Verification items for the finished model (mm, model axes). Round coordinates to 2 decimals unless told otherwise and drop trailing zeros. Loops run counter-clockwise (first coordinate to the right, second up) from the corner with the lowest first, then second, coordinate; pieces in that order, holes last.
from build123d import *

# Parameters (mm, degrees)
SKETCH1_R           = 9.625
BOSS_EXTRUDE1_DEPTH = 0.6


with BuildPart() as part:
    # Sketch1 → Boss-Extrude1 (new body)
    with BuildSketch(Plane(origin=(0, 0, 0), x_dir=(1, 0, 0), z_dir=(0, 1, 0))):
        with BuildLine():
            ThreePointArc((13.474991136, 1.1), (13.700677051, 0.553298036), (14.246293378, 0.325))
            ThreePointArc((14.246293378, 0.325), (13.165283338, 5.453238911), (10.303460358, 9.84384095))
            ThreePointArc((10.303460358, 9.84384095), (9.29660086, 9.429085476), (8.290823601, 9.846458519))
            ThreePointArc((8.290823601, 9.846458519), (8.290823601, 10.306075068), (8.750440149, 10.306075068))
            ThreePointArc((8.750440149, 10.306075068), (9.296600856, 10.079082443), (9.84384095, 10.303460358))
            ThreePointArc((9.84384095, 10.303460358), (5.453238911, 13.165283338), (0.325, 14.246293378))
            ThreePointArc((0.325, 14.246293378), (-0.09368077, 13.24105979), (-1.1, 12.824995179))
            ThreePointArc((-1.1, 12.824995179), (-1.424997978, 13.149993158), (-1.1, 13.474991136))
            ThreePointArc((-1.1, 13.474991136), (-0.553298036, 13.700677051), (-0.325, 14.246293378))
            ThreePointArc((-0.325, 14.246293378), (-5.453238911, 13.165283338), (-9.84384095, 10.303460358))
            ThreePointArc((-9.84384095, 10.303460358), (-9.429085476, 9.29660086), (-9.846458519, 8.290823601))
            ThreePointArc((-9.846458519, 8.290823601), (-10.306075068, 8.290823601), (-10.306075068, 8.750440149))
            ThreePointArc((-10.306075068, 8.750440149), (-10.079082443, 9.296600856), (-10.303460358, 9.84384095))
            ThreePointArc((-10.303460358, 9.84384095), (-13.165283338, 5.453238911), (-14.246293378, 0.325))
            ThreePointArc((-14.246293378, 0.325), (-13.24105979, -0.09368077), (-12.824995179, -1.1))
            ThreePointArc((-12.824995179, -1.1), (-13.149993158, -1.424997978), (-13.474991136, -1.1))
            ThreePointArc((-13.474991136, -1.1), (-13.700677051, -0.553298036), (-14.246293378, -0.325))
            ThreePointArc((-14.246293378, -0.325), (-13.165283338, -5.453238911), (-10.303460358, -9.84384095))
            ThreePointArc((-10.303460358, -9.84384095), (-9.29660086, -9.429085476), (-8.290823601, -9.846458519))
            ThreePointArc((-8.290823601, -9.846458519), (-8.290823601, -10.306075068), (-8.750440149, -10.306075068))
            ThreePointArc((-8.750440149, -10.306075068), (-9.296600856, -10.079082443), (-9.84384095, -10.303460358))
            ThreePointArc((-9.84384095, -10.303460358), (-5.453238911, -13.165283338), (-0.325, -14.246293378))
            ThreePointArc((-0.325, -14.246293378), (0.09368077, -13.24105979), (1.1, -12.824995179))
            ThreePointArc((1.1, -12.824995179), (1.424997978, -13.149993158), (1.1, -13.474991136))
            ThreePointArc((1.1, -13.474991136), (0.553298036, -13.700677051), (0.325, -14.246293378))
            ThreePointArc((0.325, -14.246293378), (5.453238911, -13.165283338), (9.84384095, -10.303460358))
            ThreePointArc((9.84384095, -10.303460358), (9.429085476, -9.29660086), (9.846458519, -8.290823601))
            ThreePointArc((9.846458519, -8.290823601), (10.306075068, -8.290823601), (10.306075068, -8.750440149))
            ThreePointArc((10.306075068, -8.750440149), (10.079082443, -9.296600856), (10.303460358, -9.84384095))
            ThreePointArc((10.303460358, -9.84384095), (13.165283338, -5.453238911), (14.246293378, -0.325))
            ThreePointArc((14.246293378, -0.325), (13.24105979, 0.09368077), (12.824995179, 1.1))
            ThreePointArc((12.824995179, 1.1), (13.149993158, 1.424997978), (13.474991136, 1.1))
        make_face()
        with BuildLine():
            ThreePointArc((-4.5, -11.6), (-5.1, -11), (-4.5, -10.4))
            Line((-4.5, -10.4), (4.5, -10.4))
            ThreePointArc((4.5, -10.4), (5.1, -11), (4.5, -11.6))
            Line((4.5, -11.6), (-4.5, -11.6))
        make_face(mode=Mode.SUBTRACT)
        with BuildLine():
            ThreePointArc((-11.6, 4.5), (-11, 5.1), (-10.4, 4.5))
            Line((-10.4, 4.5), (-10.4, -4.5))
            ThreePointArc((-10.4, -4.5), (-11, -5.1), (-11.6, -4.5))
            Line((-11.6, -4.5), (-11.6, 4.5))
        make_face(mode=Mode.SUBTRACT)
        with Locations(Location((0, 0, 0), (0, 0, 270))):
            Circle(SKETCH1_R, mode=Mode.SUBTRACT)
        with BuildLine():
            ThreePointArc((11.6, -4.5), (11, -5.1), (10.4, -4.5))
            Line((10.4, -4.5), (10.4, 4.5))
            ThreePointArc((10.4, 4.5), (11, 5.1), (11.6, 4.5))
            Line((11.6, 4.5), (11.6, -4.5))
        make_face(mode=Mode.SUBTRACT)
        with BuildLine():
            ThreePointArc((4.5, 11.6), (5.1, 11), (4.5, 10.4))
            Line((4.5, 10.4), (-4.5, 10.4))
            ThreePointArc((-4.5, 10.4), (-5.1, 11), (-4.5, 11.6))
            Line((-4.5, 11.6), (4.5, 11.6))
        make_face(mode=Mode.SUBTRACT)
    extrude(amount=BOSS_EXTRUDE1_DEPTH)


solid = part.part
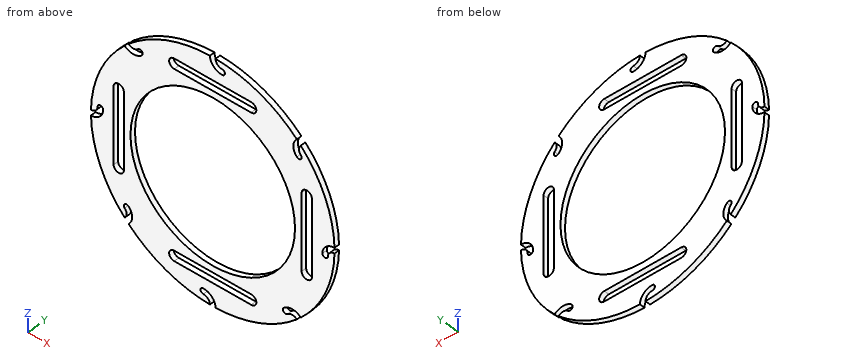
1. Section check B-B (z = -2.5). Enter the section's corners in (x, y).
2. Scan lines: L1, parallel to Z at x = 2.75, y = 0.3; L2, parallel to Z at x = 3, y = 0.1; L3, parallel to X at y = 0.4, z = -4.25. Record each from-to range of solid material in increasing order.
3. Section check C-C (y = 0.15). Give the number of separate pieces and of enclosed holes in the cut face, then the cut area to 3 significant figures.
4. Section check D-D (x = 0). Enter the section's corners in (y, z) (3 decimals).
5. Gauge pin test, flat end, axial feed: P1, Ø1.5, axis at x = 6, z = -7, coming from the -Y side. Record the tip position at first contact, or that the pin passes through.
6. Section check A-A (x = 11). Enter the section's corners in (y, z).
Taken from the geometry:
1. outline: (-14.03, 0) - (-11.6, 0) - (-11.6, 0.6) - (-14.03, 0.6) - close; (-10.4, 0) - (-9.29, 0) - (-9.29, 0.6) - (-10.4, 0.6) - close; (9.29, 0) - (10.4, 0) - (10.4, 0.6) - (9.29, 0.6) - close; (11.6, 0) - (14.03, 0) - (14.03, 0.6) - (11.6, 0.6) - close
2. L1: z = -13.98 to -11.6, -10.4 to -9.22, 9.22 to 10.4, 11.6 to 13.98
2. L2: z = -13.93 to -11.6, -10.4 to -9.15, 9.15 to 10.4, 11.6 to 13.93
2. L3: x = -13.6 to -11.6, -10.4 to -8.64, 8.64 to 10.4, 11.6 to 13.6
3. separate pieces: 1
3. enclosed holes: 5
3. area: 289 mm2
4. outline: (0, -13.344) - (0.6, -13.344) - (0.6, -11.6) - (0, -11.6) - close; (0, -10.4) - (0.6, -10.4) - (0.6, -9.625) - (0, -9.625) - close; (0, 9.625) - (0.6, 9.625) - (0.6, 10.4) - (0, 10.4) - close; (0, 11.6) - (0.6, 11.6) - (0.6, 13.344) - (0, 13.344) - close
5. P1: stops at y = 0
6. outline: (0, -9.06) - (0.6, -9.06) - (0.6, -5.1) - (0, -5.1) - close; (0, 5.1) - (0.6, 5.1) - (0.6, 9.06) - (0, 9.06) - close
